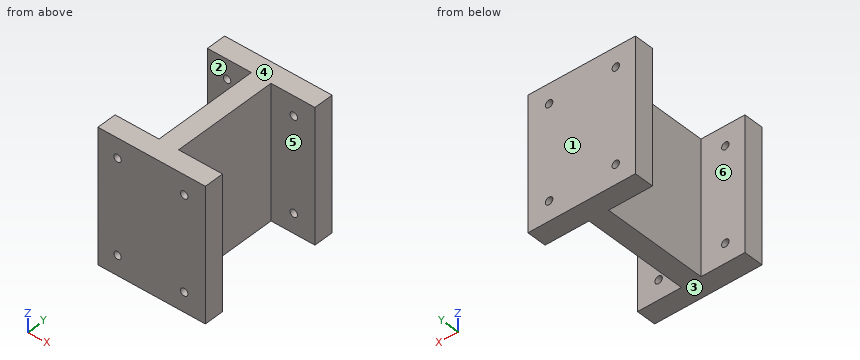
```python
from build123d import *

# Parameters (mm, degrees)
SKETCH1_W           = 34.798
SKETCH1_H           = 46.9138
BOSS_EXTRUDE1_DEPTH = 43.18
SKETCH2_W           = 14.224
SKETCH2_H           = 34.2138
CUT_EXTRUDE1_DEPTH  = 43.18
SKETCH3_R           = 1.2065
CUT_EXTRUDE2_DEPTH  = 47.9138


with BuildPart() as part:
    # Sketch1 → Boss-Extrude1 (new body)
    with BuildSketch(Plane.XY):
        with Locations((17.399, 23.4569)):
            Rectangle(SKETCH1_W, SKETCH1_H)
    extrude(amount=-BOSS_EXTRUDE1_DEPTH)

    # Sketch2 → Cut-Extrude1 (cut)
    with BuildSketch(Plane.XY):
        with Locations((7.112, 23.4569)):
            Rectangle(SKETCH2_W, SKETCH2_H)
        with Locations((27.686, 23.4569)):
            Rectangle(SKETCH2_W, SKETCH2_H)
    extrude(amount=-CUT_EXTRUDE1_DEPTH, mode=Mode.SUBTRACT)

    # Sketch3 → Cut-Extrude2 (cut, through all)
    with BuildSketch(Plane(origin=(0, 46.9138, 0), x_dir=(1, 0, 0), z_dir=(0, 1, 0))):
        with Locations((6.35, 6.35)):
            Circle(SKETCH3_R)
        with Locations((27.94, 6.35)):
            Circle(SKETCH3_R)
        with Locations((6.35, 36.83)):
            Circle(SKETCH3_R)
        with Locations((27.94, 36.83)):
            Circle(SKETCH3_R)
    extrude(amount=-CUT_EXTRUDE2_DEPTH, mode=Mode.SUBTRACT)


solid = part.part
```
The model under review builds one solid part; all positions refer to its coordinate system, in mm. Face numbers are marked on the shaded views. A direction names the side the tool comes from. Coordinates: 2 decimals unless noted, no trailing zeros. Write each loop counter-clockwise with the first axis right and the second up, starting at its lowest first coordinate (ties: lowest second). Pieces come first, ordered by that corner, then holes. Notation, with made-up numbers: (32.5, -21.75) -> (83.5, -21.75) arc R31 cw to (83.5, 16.25) -> close; hole circle Ø7 at (65, 23.25). An arc over 180 degrees is marked (long way). One line per item, written item: value. Start each with the question number.
Q1. Clearance check with flat-ended pins moving along their axes: P1, Ø3, axis at x = 17, z = -7, coming from the -Y side; P2, Ø4, axis at y = 17.5, z = -26.5, coming from the +X side. State where each tip first meets the part, or that it passes through.
Q2. For the marked faces 4, 5 and 6, list the 3-axis set-ups (+Z, -Z, +X, -X, +Y, -Y) from which the entire face can be reached by the end or side of a thin tool; tool diameter is ignored.
Q3. The part is to be moulded in two halves that separate along Y. For the marked faces 1, 2 and 3, say which applies: +Y half, -Y half, draft (parallel to the pull), parting line (faces both ways), or undercut.
Q4. Add section D-D, the plane z = -30.5. Give the boundary of the cut face in (x, y).
Q5. Add section B-B, the plane z = -36.83. Give the boundary of the cut face in (x, y), then the cut area to 3 significant figures.
Q6. Add section C-C, the plane x = 21.5. Give the boundary of the cut face in (y, z).
Q7. To check wall thickness, follow probe 1 along Z at (x, y) = (27.94, 3.25); probe 2 along X at (y, z) = (43.5, -6.35); probe 3 along Y at (x, z) = (26, -16.5). State the ranges of each line that lie inside material, in increasing order.
Q8. Add section A-A, the plane x = 6.35. Give the boundary of the cut face in (y, z), then the cut area to 3 significant figures.
Response:
1. P1: y = 0
1. P2: x = 20.57
2. face 4: +Z, +X, -X, +Y, -Y
2. face 5: +Z, -Z, +X
2. face 6: +Z, -Z, -X
3. face 1: +Y half
3. face 2: undercut
3. face 3: draft
4. outline: (0, 0) -> (34.8, 0) -> (34.8, 6.35) -> (20.57, 6.35) -> (20.57, 40.56) -> (34.8, 40.56) -> (34.8, 46.91) -> (0, 46.91) -> (0, 40.56) -> (14.22, 40.56) -> (14.22, 6.35) -> (0, 6.35) -> close
5. outline: (0, 0) -> (5.14, 0) -> (5.14, 6.35) -> (0, 6.35) -> close; (0, 40.56) -> (5.14, 40.56) -> (5.14, 46.91) -> (0, 46.91) -> close; (7.56, 0) -> (26.73, 0) -> (26.73, 6.35) -> (20.57, 6.35) -> (20.57, 40.56) -> (26.73, 40.56) -> (26.73, 46.91) -> (7.56, 46.91) -> (7.56, 40.56) -> (14.22, 40.56) -> (14.22, 6.35) -> (7.56, 6.35) -> close; (29.15, 0) -> (34.8, 0) -> (34.8, 6.35) -> (29.15, 6.35) -> close; (29.15, 40.56) -> (34.8, 40.56) -> (34.8, 46.91) -> (29.15, 46.91) -> close
5. area: 598 mm²
6. outline: (0, -43.18) -> (6.35, -43.18) -> (6.35, 0) -> (0, 0) -> close; (40.56, -43.18) -> (46.91, -43.18) -> (46.91, 0) -> (40.56, 0) -> close
7. probe 1: -43.18 to -38.04, -35.62 to -7.56, -5.14 to 0
7. probe 2: 0 to 5.14, 7.56 to 26.73, 29.15 to 34.8
7. probe 3: 0 to 6.35, 40.56 to 46.91
8. outline: (0, -43.18) -> (6.35, -43.18) -> (6.35, -38.04) -> (0, -38.04) -> close; (0, -35.62) -> (6.35, -35.62) -> (6.35, -7.56) -> (0, -7.56) -> close; (0, -5.14) -> (6.35, -5.14) -> (6.35, 0) -> (0, 0) -> close; (40.56, -43.18) -> (46.91, -43.18) -> (46.91, -38.04) -> (40.56, -38.04) -> close; (40.56, -35.62) -> (46.91, -35.62) -> (46.91, -7.56) -> (40.56, -7.56) -> close; (40.56, -5.14) -> (46.91, -5.14) -> (46.91, 0) -> (40.56, 0) -> close
8. area: 487 mm²
